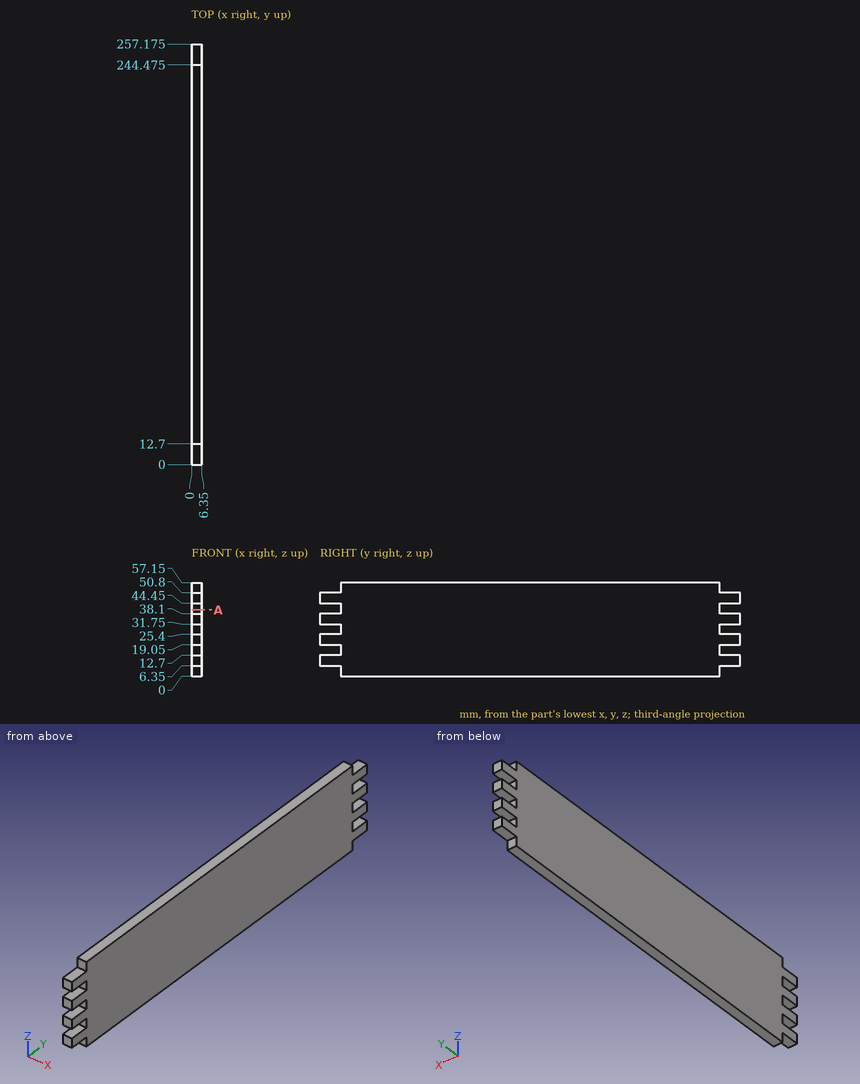
Print and shaded views of the part. All mm, measured from the part's lowest x, y and z. Coordinates: 2 decimals unless noted, no trailing zeros. Write each loop counter-clockwise with the first axis right and the second up, starting at its lowest first coordinate (ties: lowest second). Pieces come first, ordered by that corner, then holes.
(1) Drill centre line: probe 1 along Y at (x, z) = (0.5, 31.5) (3 decimals). Where is it in solid material? Low to high.
(2) Flat gauge pins, fed straight in: pin 1 (3 mm diameter, centred on x = 1.5, y = 8.5, fed in from +Z); pin 2 (6 mm diameter, centred on y = 140, z = 37.5, fed in from -X); pin 3 (1.9 mm diameter, centred on x = 3.5, z = 14.5, fed in from +Y) (3 decimals); pin 4 (1.9 mm diameter, centred on x = 3.5, z = 55, fed in from -Y). Where does each tip first touch, or does it go through?
(3) Cut at A-A, the plane z = 40.5. List the corners of the cut face in (x, y) (3 decimals), and give its area (3 significant figures).
Geometry says:
1. probe 1: y = 12.7 to 244.475
2. pin 1: stops at z = 50.8
2. pin 2: stops at x = 0
2. pin 3: stops at y = 244.475
2. pin 4: stops at y = 12.7
3. outline: (0, 12.7) - (6.35, 12.7) - (6.35, 244.475) - (0, 244.475) - close
3. area: 1,470 mm2
